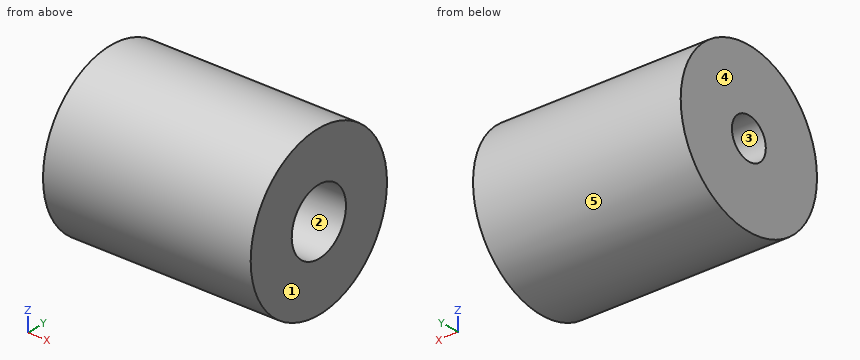
Autodesk Inventor part; units mm, degrees
ref_plane "YZ Plane" through (0, 0, 0) normal (1, 0, 0) x (0, 1, 0)
ref_plane "XZ Plane" through (0, 0, 0) normal (0, 1, 0) x (-1, 0, 0)
ref_plane "XY Plane" through (0, 0, 0) normal (0, 0, 1) x (1, 0, 0)
sketch "Sketch1" plane through (0, 0, 0) normal (1, 0, 0) x (0, 1, 0)
  circle A0 centre (0, 0) radius 10.05
  dimension "d0" = 20.1
extrude "Extrusion1" add sketch "Sketch1" along normal mid plane 25.45
sketch "Sketch2" plane through (12.725, 0, 0) normal (1, 0, 0) x (0, 0, -1)
  circle A0 centre (0, 0) radius 4
  dimension "d3" = 8
hole "Hole1" at (12.725, 0, 0) direction (-1, 0, 0) diameter 8 depth 16.57
sketch "Sketch3" plane through (-12.725, 0, 0) normal (-1, 0, 0) x (0, 0, 1)
  circle A0 centre (0, 0) radius 2.5
  dimension "d11" = 5
hole "Hole2" at (-12.725, 0, 0) direction (1, 0, 0) diameter 5 end through all
properties part number "CNC-1.1v-S-1-( thread coupler)"
Check sheet for the modelled part. Datum: model origin and axes. Units: mm. Face numbers are marked on the shaded views. A direction names the side the tool comes from. Round coordinates to 2 decimals unless told otherwise and drop trailing zeros. Loops run counter-clockwise (first coordinate to the right, second up) from the corner with the lowest first, then second, coordinate; pieces in that order, holes last. Notation, with made-up numbers: (42.5, -35.5) -> (71.5, -35.5) arc R12 ccw to (71.5, -15.5) -> close; hole circle Ø3 at (84, -29). An arc over 180 degrees is marked (long way). Put each result on its own line as item: value. Start each with the question number.
1. Scan lines: probe 1 along Z at (x, y) = (-7.5, 0); probe 2 along Z at (x, y) = (9, 0); probe 3 along Y at (x, z) = (5.75, 0.5). Record each from-to range of solid material in increasing order.
2. Section check A-A (z = 0). Enter the section's corners in (x, y) (3 decimals), plus the area to 3 significant figures.
3. Draft check along Y on the marked faces 3, 4 and 5. Enter one of: +Y half, -Y half, draft (parallel to the pull), parting line (faces both ways), or undercut.
4. Section check C-C (x = 0). Enter the section's corners in (y, z).
5. Gauge pin test, flat ends, axial feed: pin 1 (4 mm diameter, centred on y = 0, z = 0, fed in from +X); pin 2 (10 mm diameter, centred on x = 10, y = 6, fed in from -Z); pin 3 (5 mm diameter, centred on x = 5.5, z = 3.5, fed in from -Y); pin 4 (2 mm diameter, centred on x = -2.5, z = 7, fed in from -Y). Record the tip position at first contact, or that the pin passes through.
6. Section check D-D (z = 3.5). Enter the section's corners in (x, y) (1 decimal).
7. Access from +Z, -Z, +X, -X, +Y, -Y to the whole of each face (thin tool, end or side, straight path). Record for the marked faces 1 and 2.
Findings:
1. probe 1: z = -10.05 to -2.5, 2.5 to 10.05
1. probe 2: z = -10.05 to -4, 4 to 10.05
1. probe 3: y = -10.04 to -3.97, 3.97 to 10.04
2. outline: (-12.725, -10.05) -> (12.725, -10.05) -> (12.725, -4) -> (-3.845, -4) -> (-3.845, -2.5) -> (-12.725, -2.5) -> close; (-12.725, 2.5) -> (-3.845, 2.5) -> (-3.845, 4) -> (12.725, 4) -> (12.725, 10.05) -> (-12.725, 10.05) -> close
2. area: 335 mm^2
3. face 3: undercut
3. face 4: draft
3. face 5: parting line
4. outline: circle Ø20.1 at (0, 0); hole circle Ø8 at (0, 0)
5. pin 1: passes through
5. pin 2: stops at z = -10
5. pin 3: stops at y = -10
5. pin 4: stops at y = -8.06
6. outline: (-12.7, -9.4) -> (12.7, -9.4) -> (12.7, -1.9) -> (-3.8, -1.9) -> (-3.8, 1.9) -> (12.7, 1.9) -> (12.7, 9.4) -> (-12.7, 9.4) -> close
7. face 1: +Z, -Z, +X, +Y, -Y
7. face 2: +X
